```python
from build123d import *

# Parameters (mm, degrees)
BOSS_EXTRUDE1_DEPTH   = 15.24
F_8_0MM_DOWEL_HOLE1_D = 8
SKETCH5_W             = 5.08
SKETCH5_H             = 101.6
CUT_EXTRUDE1_DEPTH    = 87.135590786


with BuildPart() as part:
    # Sketch1 → Boss-Extrude1 (new body)
    with BuildSketch(Plane(origin=(0, 0, 0), x_dir=(0, 0, -1), z_dir=(1, 0, 0))):
        with BuildLine():
            Line((-77.47, 8.41375), (49.53, 8.41375))
            ThreePointArc((49.53, 8.41375), (55.88, 2.06375), (49.53, -4.28625))
            Line((49.53, -4.28625), (-77.47, -4.28625))
            ThreePointArc((-77.47, -4.28625), (-83.82, 2.06375), (-77.47, 8.41375))
        make_face()
    extrude(amount=BOSS_EXTRUDE1_DEPTH)

    # Ø8.0mm Dowel Hole1 (through all)
    with Locations(Plane(origin=(15.24, 0, 0), x_dir=(0, 0, -1), z_dir=(1, 0, 0))):
        with Locations((-77.47, 2.06375), (49.53, 2.06375), (-13.97, 2.06375)):
            Hole(F_8_0MM_DOWEL_HOLE1_D / 2)

    # Sketch5 → Cut-Extrude1 (cut, through all)
    with BuildSketch(Plane(origin=(0, 8.41375, 0), x_dir=(1, 0, 0), z_dir=(0, 1, 0))):
        with Locations((7.62, -13.97)):
            Rectangle(SKETCH5_W, SKETCH5_H)
    extrude(amount=-CUT_EXTRUDE1_DEPTH, mode=Mode.SUBTRACT)


solid = part.part
```
The model under review builds one solid part; all positions refer to its coordinate system, in mm. A direction names the side the tool comes from. Coordinates: 2 decimals unless noted, no trailing zeros. Write each loop counter-clockwise with the first axis right and the second up, starting at its lowest first coordinate (ties: lowest second). Pieces come first, ordered by that corner, then holes.
1) The part is to be moulded in two halves that separate along Z. For faces 1 (the face through (7.513, 2.24, 73.474)), 2 (the face through (12.664, 2.24, 9.974)), 3 (the face through (7.51, 1.92, 83.82)), 4 (the face through (15.24, -2, 13)), say which applies: pulls with the +Z half, pulls with the -Z half, needs draft (parallel to the pull), parting line crosses it, or undercut.
2) We need section D-D on x = 13.25. State the section outline as (y, z) points, then the cut area to 3 significant figures.
3) We need section A-A on z = 13.97. State the section outline as (x, y) points.
4) We need section B-B on z = 42. State the section outline as (x, y) points, then the cut area to 3 significant figures.
5) Machinability: for faces 5 (the face through (7.51, 2.2, -55.88)), 6 (the face through (8, 2, 64.77)), which of the approach directions +Z, -Z, +X, -X, +Y, -Y give a long, thin tool a straight path to every point of the face, cutting with its end or side? Answer none if there is none.
6) Clearance check with flat-ended pins moving along their axes: pin 1 Ø5.5 at (x, y) = (9, 0.5) entering from +Z; pin 2 Ø3 at (x, y) = (5, -3) entering from +Z; pin 3 Ø5 at (y, z) = (2.06, 13.97) entering from -X; pin 4 Ø5.5 at (x, y) = (9, 5) entering from -Z. State where each tip first meets the part, or that it passes through.
7) We need section C-C on x = 7. State the section outline as (y, z) points, then the cut area to 3 significant figures.
8) To check wall thickness, follow probe 1 along Z at (x, y) = (7.25, 2.5) (3 decimals); probe 2 along Z at (x, y) = (8.5, 2.25); probe 3 along X at (y, z) = (7, 62). State the ranges of each line that lie inside material, in increasing order.
Answer list:
1. face 1: undercut
1. face 2: undercut
1. face 3: pulls with the +Z half
1. face 4: needs draft
2. outline: (-4.29, -49.53) arc R6.35 ccw to (8.41, -49.53) - (8.41, 77.47) arc R6.35 ccw to (-4.29, 77.47) - close; hole circle Ø8 at (2.06, -49.53); hole circle Ø8 at (2.06, 13.97); hole circle Ø8 at (2.06, 77.47)
2. area: 1,590 mm2
3. outline: (0, -4.29) - (5.08, -4.29) - (5.08, -1.94) - (0, -1.94) - close; (0, 6.06) - (5.08, 6.06) - (5.08, 8.41) - (0, 8.41) - close; (10.16, -4.29) - (15.24, -4.29) - (15.24, -1.94) - (10.16, -1.94) - close; (10.16, 6.06) - (15.24, 6.06) - (15.24, 8.41) - (10.16, 8.41) - close
4. outline: (0, -4.29) - (5.08, -4.29) - (5.08, 8.41) - (0, 8.41) - close; (10.16, -4.29) - (15.24, -4.29) - (15.24, 8.41) - (10.16, 8.41) - close
4. area: 129 mm2
5. face 5: -Z, +X, -X
5. face 6: +Y, -Y
6. pin 1: stops at z = 83.82
6. pin 2: stops at z = 82.73
6. pin 3: passes through
6. pin 4: stops at z = -55.88
7. outline: (-4.29, -49.53) arc R6.35 ccw to (8.41, -49.53) - (8.41, -36.83) - (-4.29, -36.83) - close; (-4.29, 64.77) - (8.41, 64.77) - (8.41, 77.47) arc R6.35 ccw to (-4.29, 77.47) - close; hole circle Ø8 at (2.06, -49.53); hole circle Ø8 at (2.06, 77.47)
7. area: 349 mm2
8. probe 1: z = -55.865 to -53.506, -45.554 to -36.83, 64.77 to 73.494, 81.446 to 83.805
8. probe 2: z = -55.88 to -53.53, -45.53 to -36.83, 64.77 to 73.47, 81.47 to 83.82
8. probe 3: x = 0 to 5.08, 10.16 to 15.24
